Check sheet for the modelled part. Datum: model origin and axes. Units: mm. A direction names the side the tool comes from. Round coordinates to 2 decimals unless told otherwise and drop trailing zeros. Order: outer loops, then holes, each group sorted by start corner. A loop starts at its lowest first (then second) coordinate and runs counter-clockwise, first axis right, second up. Notation, with made-up numbers: (-12, 70.5) -> (21, 70.5) arc R22 cw to (21, 82.5) -> close; hole circle Ø10 at (42, 4). An arc over 180 degrees is marked (long way). Use CSV: the item, a comma, the result in double quotes.
Autodesk Inventor part; units mm, degrees
ref_plane "YZ Plane" through (0, 0, 0) normal (1, 0, 0) x (0, 1, 0)
ref_plane "XZ Plane" through (0, 0, 0) normal (0, 1, 0) x (-1, 0, 0)
ref_plane "XY Plane" through (0, 0, 0) normal (0, 0, 1) x (1, 0, 0)
sketch "Sketch1" plane through (0, 0, 0) normal (0, 0, 1) x (1, 0, 0)
  line L0 (-10.627, -30.5907) -> (-13.477, -30.5907)
  line L1 (-10.627, -30.5907) -> (-10.627, -50.5907)
  line L2 (-10.627, -50.5907) -> (-12.127, -50.5907)
  line L3 (-12.127, -50.5907) -> (-12.127, -30.5907)
  line L4 (-10.627, -30.5907) -> (-10.627, -26.5988)
  line L5 (-13.477, -30.5907) -> (-13.477, -30.2107)
  line L6 (-13.477, -30.2107) -> (-13.477, -28.9407)
  line L7 (-13.477, -28.9407) -> (-10.627, -28.9407)
  dimension "d0" = 2.85
  dimension "d2" = 20
  dimension "d3" = 1.5
  dimension "d18" = 0.38
  dimension "d19" = 1.65
revolve "Revolution1" add sketch "Sketch1" angle 360 about axis through (-10.627, -30.5907, 0) along (0, -1, 0)
chamfer "Chamfer2" distance 0.2 angle 45 1 edges at (-9.127, -50.5907, 0)
fillet "Empalme2" radius 1.27 1 edges at (-7.777, -28.9407, 0)
sketch "Boceto2" plane through (-10.627, -28.9407, 0) normal (0, 1, 0) x (1, 0, 0)
  line L0 (0.8985, 0.7252) -> (1.0773, -0.4156)
  line L1 (1.0773, -0.4156) -> (0.1788, -1.1408)
  line L2 (0.1788, -1.1408) -> (-0.8985, -0.7252)
  line L3 (-0.8985, -0.7252) -> (-1.0773, 0.4156)
  line L4 (-1.0773, 0.4156) -> (-0.1788, 1.1408)
  line L5 (-0.1788, 1.1408) -> (0.8985, 0.7252)
  point P0 (10.627, 0)
  point P1 (0, 0)
  dimension "d21" = 2
extrude "Extrusión1" cut sketch "Boceto2" against normal blind 1.3
thread "Rosca2"
properties part number "Tornillo Allen cabeeza botón M3x20mm"
Q1. Scan lines: L1, parallel to Y at x = -10.1, z = -0.65; L2, parallel to Y at x = -10.8, z = -1.6; L3, parallel to Z at x = -11.6, y = -41. Record each from-to range of solid material in increasing order.
Result sheet:
L1,"y = -50.59 to -30.24"
L2,"y = -30.59 to -28.94"
L3,"z = -1.14 to 1.14"
Q2. Access from +Z, -Z, +X, -X, +Y, -Y to the whole of each face (thin tool, end or side, straight path). Record for faces 4 (the face through (-12, -28.941, 0)), 5 (the face through (-12, -30.591, 1)), 6 (the face through (-10.979, -29.582, 0.936)).
Result sheet:
face 4,"+Z, -Z, +X, -X, +Y"
face 5,"-Y"
face 6,"+Y"
Q3. Sectioned sample at A-A, the plane z = 0. Enter the section's corners in (x, y), then the cut area to 3 significant figures.
Result sheet:
outline,"(-13.48, -30.59) -> (-12.13, -30.59) -> (-12.13, -50.39) -> (-11.93, -50.59) -> (-9.33, -50.59) -> (-9.13, -50.39) -> (-9.13, -30.59) -> (-7.78, -30.59) -> (-7.78, -30.21) arc R1.27 ccw to (-9.05, -28.94) -> (-9.61, -28.94) -> (-9.61, -30.24) -> (-11.64, -30.24) -> (-11.64, -28.94) -> (-12.21, -28.94) arc R1.27 ccw to (-13.48, -30.21) -> close"
area,"66.0 mm^2"
Q4. Mould release check, pull along Z, two halves, no side actions. Record for faces 1 (the face through (-13.26, -30.4, -1.09)), 2 (the face through (-10.275, -29.582, -0.936)), 3 (the face through (-11, -50.591, 0)): pulls with the +Z half, pulls with the -Z half, needs draft (parallel to the pull), parting line crosses it, or undercut.
Result sheet:
face 1,"parting line crosses it"
face 2,"undercut"
face 3,"needs draft"
Q5. Go/stop test with flat-tipped pins: pin 1 (2 mm diameter, centred on x = -12.5, z = -2, fed in from -Y); pin 2 (1.5 mm diameter, centred on x = -8.5, z = -2, fed in from +Y); pin 3 (2 mm diameter, centred on y = -42, z = -0.5, fed in from -X). Record where each tip stops, or that it passes through.
Result sheet:
pin 1,"stops at y = -30.59"
pin 2,"stops at y = -29.09"
pin 3,"stops at x = -12.13"
Q6. Sectioned sample at B-B, the plane y = -34.25. Enter the section's corners in (x, z).
Result sheet:
outline,"circle Ø3 at (-10.63, 0)"
